Work out the finished part from the listing and answer in its coordinate system (mm). A direction names the side the tool comes from. Round coordinates to 2 decimals unless told otherwise and drop trailing zeros. Loops run counter-clockwise (first coordinate to the right, second up) from the corner with the lowest first, then second, coordinate; pieces in that order, holes last.
```python
from build123d import *

# Parameters (mm, degrees)
SKETCH1_R           = 45
SKETCH1_R_2         = 30
BOSS_EXTRUDE1_DEPTH = 20
SKETCH2_W           = 40
SKETCH2_H           = 80
BOSS_EXTRUDE2_DEPTH = 20
SKETCH3_W           = 40
SKETCH3_H           = 20
BOSS_EXTRUDE3_DEPTH = 20
FILLET1_R           = 2.5
SKETCH4_R           = 4
CUT_EXTRUDE1_DEPTH  = 21


with BuildPart() as part:
    # Sketch1 → Boss-Extrude1 (new body)
    with BuildSketch(Plane(origin=(0, 0, 0), x_dir=(1, 0, 0), z_dir=(0, 1, 0))):
        Circle(SKETCH1_R)
        Circle(SKETCH1_R_2, mode=Mode.SUBTRACT)
    extrude(amount=BOSS_EXTRUDE1_DEPTH)

    # Sketch2 → Boss-Extrude2 (add)
    with BuildSketch(Plane(origin=(0, 0, 0), x_dir=(1, 0, 0), z_dir=(0, 1, 0))):
        with Locations((0, 70)):
            Rectangle(SKETCH2_W, SKETCH2_H)
    extrude(amount=BOSS_EXTRUDE2_DEPTH)

    # Sketch3 → Boss-Extrude3 (add)
    with BuildSketch(Plane(origin=(0, 20, 0), x_dir=(1, 0, 0), z_dir=(0, 1, 0))):
        with Locations((0, 100)):
            Rectangle(SKETCH3_W, SKETCH3_H)
    extrude(amount=BOSS_EXTRUDE3_DEPTH)

    # Fillet1
    fillet1_edges = [part.edges().sort_by_distance(p)[0] for p in [
        (0, 20, -90),
    ]]
    fillet(fillet1_edges, radius=FILLET1_R)

    # Sketch4 → Cut-Extrude1 (cut, through all)
    with BuildSketch(Plane.XY.offset(-90)):
        with Locations((10, 31)):
            Circle(SKETCH4_R)
        with Locations((-10, 31)):
            Circle(SKETCH4_R)
    extrude(amount=-CUT_EXTRUDE1_DEPTH, mode=Mode.SUBTRACT)


solid = part.part
```
1. Find section A-A (x = 0). Write down the section's boundary in (y, z), then the cut area to 3 significant figures.
Answer key:
outline: (0, -110) - (40, -110) - (40, -90) - (22.5, -90) arc R2.5 cw to (20, -87.5) - (20, -30) - (0, -30) - close; (0, 30) - (20, 30) - (20, 45) - (0, 45) - close
area: 2,300 mm2
2. Find section D-D (z = -95). Write down the section's boundary in (x, y).
Answer key:
outline: (-20, 0) - (20, 0) - (20, 40) - (-20, 40) - close; hole circle Ø8 at (-10, 31); hole circle Ø8 at (10, 31)
3. Determine the mould class of faces 1 (the face through (0, 40, -100)), 2 (the face through (-29.97, 9.86, -1.32)), 3 (the face through (0, 31, -90)), 4 (the face through (0, 20, -110)) for opening direction Z: +Z half, -Z half, draft (parallel to the pull), parting line (faces both ways), or undercut.
Answer key:
face 1: draft
face 2: undercut
face 3: +Z half
face 4: -Z half
4. Find section C-C (y = 31). Write down the section's boundary in (x, z), then the cut area to 3 significant figures.
Answer key:
outline: (-20, -110) - (-14, -110) - (-14, -90) - (-20, -90) - close; (-6, -110) - (6, -110) - (6, -90) - (-6, -90) - close; (14, -110) - (20, -110) - (20, -90) - (14, -90) - close
area: 480 mm2
5. Consider probe 1 along Z at (x, y) = (0, 8); probe 2 along Y at (x, z) = (-10, -100.5); probe 3 along X at (y, z) = (10, 0). Determine where each line is inside the solid, lowest interval first.
Answer key:
probe 1: z = -110 to -30, 30 to 45
probe 2: y = 0 to 27, 35 to 40
probe 3: x = -45 to -30, 30 to 45
6. Find section B-B (z = 0). Write down the section's boundary in (x, y).
Answer key:
outline: (-45, 0) - (-30, 0) - (-30, 20) - (-45, 20) - close; (30, 0) - (45, 0) - (45, 20) - (30, 20) - close
7. Which of the six approach directions +Z, -Z, +X, -X, +Y, -Y give full straight-line access (tool end or side, diameter ignored) to faces 5 (the face through (-20, 15, -82)), 6 (the face through (-1, 20, -37)), 7 (the face through (20, 15, -82)), 8 (the face through (9.479, 34.966, -99.86))?
Answer key:
face 5: -Z, -X, +Y, -Y
face 6: +Z, +X, -X, +Y
face 7: -Z, +X, +Y, -Y
face 8: +Z, -Z
8. Given pin 1 (4 mm diameter, centred on y = 12.5, z = -86.5, fed in from +X); pin 2 (20 mm diameter, centred on y = 15.5, z = -61, fed in from -X); pin 3 (4 mm diameter, centred on x = 31.5, z = -18.5, fed in from +Y), each flat-ended and moving along its own axis, determine where each tip first touches the part or whether it passes through.
Answer key:
pin 1: stops at x = 20
pin 2: stops at x = -20
pin 3: stops at y = 20
